Source: three-view drawing plus pictorial views. Frame: mm from the lowest corner of the part. Give positions to 0.01 mm unless a question says otherwise; leave off trailing zeros. Order: outer loops, then holes, each group sorted by start corner. A loop starts at its lowest first (then second) coordinate and runs counter-clockwise, first axis right, second up. Notation, with made-up numbers: (-33, -13.75) - (20, -13.75) arc R16 cw to (20, -7.75) - close; hole circle Ø11 at (76.25, -25). An arc over 180 degrees is marked (long way). Answer in a Markdown table with one row per item. Add a question column.
1. Section query C-C on z = 1.25. Return loops of the section in (x, y).
2. Ray query, line 1 (Y direction, x = 14, z = 0.2); line 2 (Y direction, x = 15, z = 0.65); line 3 (X direction, y = 16.5, z = 2.35). Return the intervals inside material, ascending. Write a range as [from, to].
3. Section query A-A on x = 14. Return loops of the section in (y, z).
4. Contact query for flat-ended pins moving along their axis: pin 1 (1.5 mm diameter, centred on x = 6.5, y = 10.5, fed in from -Z); pin 2 (5 mm diameter, centred on x = 14, y = 14, fed in from +Z); pin 3 (1.5 mm diameter, centred on x = 12, z = 2, fed in from +Y). Output: stop coordinate, or through.
5. Mould query, pull axis Y, two halves, no side actions, for the marked faces 1, 2 and 3. Classes: released by +Y, released by -Y, zero draft, split by the parting line, or undercut.
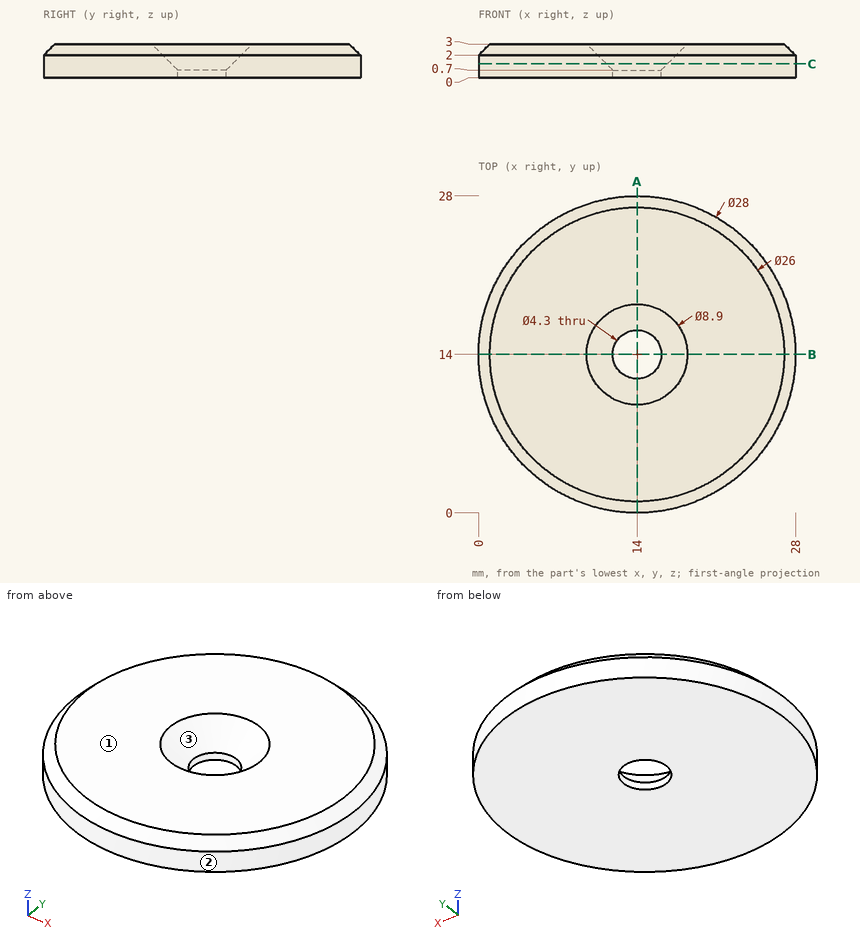
Answer:
| question | item | result |
|---|---|---|
| 1 | outline | circle Ø28 at (14, 14); hole circle Ø5.4 at (14, 14) |
| 2 | line 1 | y = [0, 11.85], [16.15, 28] |
| 2 | line 2 | y = [0.04, 12.1], [15.9, 27.96] |
| 2 | line 3 | x = [0.58, 11.14], [16.86, 27.42] |
| 3 | outline | (0, 0) - (11.85, 0) - (11.85, 0.7) - (9.55, 3) - (1, 3) - (0, 2) - close; (16.15, 0) - (28, 0) - (28, 2) - (27, 3) - (18.45, 3) - (16.15, 0.7) - close |
| 4 | pin 1 | stops at z = 0 |
| 4 | pin 2 | stops at z = 1.05 |
| 4 | pin 3 | stops at y = 27.94 |
| 5 | face 1 | zero draft |
| 5 | face 2 | split by the parting line |
| 5 | face 3 | undercut |
